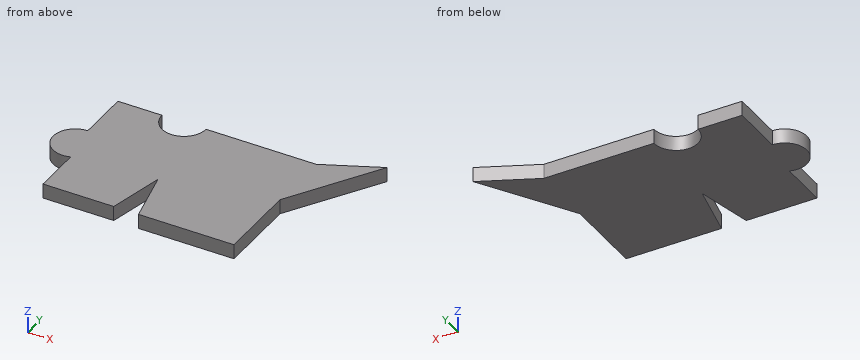
```python
from build123d import *

# Parameters (mm, degrees)
PAD_DEPTH = 10


with BuildPart() as part:
    # Sketch → Pad (new body)
    with BuildSketch(Plane.XY):
        with BuildLine():
            Line((111.489324, 77.916617), (73.424397, 60.16665))
            Line((73.424397, 60.16665), (-1.575603, 60.16665))
            ThreePointArc((-31.575603, 60.16665), (-16.575603, 45.16665), (-1.575603, 60.16665))
            Line((-31.575603, 60.16665), (-61.575603, 60.16665))
            Line((-61.575603, 60.16665), (-61.575603, 24.16665))
            ThreePointArc((-61.575603, 24.16665), (-76.359581, 6.63012), (-56.575603, -4.975486))
            Line((-56.575603, -4.975486), (-56.575603, -38))
            Line((-56.575603, -38), (-8.424397, -38))
            Line((-8.424397, -38), (0, 0))
            Line((0, 0), (8.424397, -38))
            Line((8.424397, -38), (73.424397, -38))
            Line((73.424397, -38), (73.424397, 17))
            Line((73.424397, 17), (111.489324, 77.916617))
        make_face()
    extrude(amount=PAD_DEPTH)


solid = part.part
```
CAD build for the part. Positions are in the model's coordinates, mm. Give positions to 0.01 mm unless a question says otherwise; leave off trailing zeros. Loops run counter-clockwise (first coordinate to the right, second up) from the corner with the lowest first, then second, coordinate; pieces in that order, holes last. Notation, with made-up numbers: (21.25, 32) - (65.25, 32) arc R38 ccw to (65.25, 70) - close; hole circle Ø4 at (52.5, 1). An arc over 180 degrees is marked (long way). Put each result on its own line as item: value.
Q1. Slice it at D-D (y = 51.5). Give the cut face in (x, z), plus the area to 3 significant figures.
Filled in:
outline: (-61.58, 0) - (-28.82, 0) - (-28.82, 10) - (-61.58, 10) - close; (-4.33, 0) - (94.98, 0) - (94.98, 10) - (-4.33, 10) - close
area: 1,320 mm²
Q2. Probe line 1 along Y through (x, z) = (39, 4.75); line 2 along X through (y, z) = (-14, 6.75); line 3 along Y through (x, z) = (75.5, 1.75). List the from-to ranges inside material, lowest first.
Filled in:
line 1: y = -38 to 60.17
line 2: x = -56.58 to -3.1, 3.1 to 73.42
line 3: y = 20.32 to 61.13
Q3. Slice it at A-A (z = 6). Give the cut face in (x, y), plus the area to 3 significant figures.
Filled in:
outline: (-61.58, 24.17) arc R15 ccw (long way) to (-56.58, -4.98) - (-56.58, -38) - (-8.42, -38) - (0, 0) - (8.42, -38) - (73.42, -38) - (73.42, 17) - (111.49, 77.92) - (73.42, 60.17) - (-1.58, 60.17) arc R15 cw to (-31.58, 60.17) - (-61.58, 60.17) - close
area: 13,600 mm²
Q4. Flat gauge pins, fed straight in: pin 1 (3 mm diameter, centred on x = -46.5, z = 7, fed in from +Y); pin 2 (5 mm diameter, centred on y = 41, z = 6, fed in from -X); pin 3 (3 mm diameter, centred on y = -16, z = 7, fed in from -X). Where does each tip first touch, or does it go through?
Filled in:
pin 1: stops at y = 60.17
pin 2: stops at x = -61.58
pin 3: stops at x = -56.58
Q5. Slice it at C-C (x = 31). Give the cut face in (y, z).
Filled in:
outline: (-38, 0) - (60.17, 0) - (60.17, 10) - (-38, 10) - close
Q6. Slice it at B-B (y = -24.5). Give the cut face in (x, z), plus the area to 3 significant figures.
Filled in:
outline: (-56.58, 0) - (-5.43, 0) - (-5.43, 10) - (-56.58, 10) - close; (5.43, 0) - (73.42, 0) - (73.42, 10) - (5.43, 10) - close
area: 1,190 mm²
